Read the model definition and answer for the solid it produces. Units are mm, in the model's axes. A direction names the side the tool comes from. Give positions to 0.01 mm unless a question says otherwise; leave off trailing zeros. Order: outer loops, then holes, each group sorted by start corner. A loop starts at its lowest first (then second) coordinate and runs counter-clockwise, first axis right, second up. Notation, with made-up numbers: (-27, -22) - (2, -22) arc R24 ccw to (2, 10) - close; hole circle Ø10 at (71, -2). An arc over 180 degrees is marked (long way). Write item = value, one per line.
```python
from build123d import *

# Parameters (mm, degrees)
PAD_DEPTH         = 50
SKETCH001_R       = 20
POCKET_DEPTH      = 50.001
POCKET_DEPTH_BACK = 0.001
PAD001_DEPTH      = 10
SKETCH003_W       = 200
SKETCH003_H       = 125
PAD002_DEPTH      = 50
SKETCH004_W       = 25
SKETCH004_H       = 75
POCKET001_DEPTH   = 200.001
POCKET002_DEPTH   = 40


with BuildPart() as part:
    # Sketch → Pad (new body)
    with BuildSketch(Plane.XZ):
        with BuildLine():
            Line((-35, -35), (35, -35))
            Line((35, -35), (35, 0))
            ThreePointArc((35, 0), (0, 35), (-35, 0))
            Line((-35, 0), (-35, -35))
        make_face()
    extrude(amount=PAD_DEPTH)

    # Sketch001 (on Face6 of Pad) → Pocket (cut, two sides)
    with BuildSketch(Plane.XZ.offset(50)) as pocket_sk:
        Circle(SKETCH001_R)
    extrude(amount=-POCKET_DEPTH, mode=Mode.SUBTRACT)
    extrude(pocket_sk.sketch, amount=POCKET_DEPTH_BACK, mode=Mode.SUBTRACT)

    # Sketch002 (on Face5 of Pocket) → Pad001 (join)
    with BuildSketch(Plane.XZ.offset(50)):
        Polygon((35, -35), (95, -35), (22.707273, 26.634184), align=None)
    extrude(amount=-PAD001_DEPTH)

    # Sketch003 (on Face8 of Pad001) → Pad002 (join)
    with BuildSketch(Plane(origin=(0, 0, -35), x_dir=(1, 0, 0), z_dir=(0, 0, -1))):
        with Locations((65, -12.5)):
            Rectangle(SKETCH003_W, SKETCH003_H)
    extrude(amount=PAD002_DEPTH)

    # Sketch004 (on Face10 of Pad002) → Pocket001 (cut, through all)
    with BuildSketch(Plane(origin=(165, 0, 0), x_dir=(0, 0, 1), z_dir=(1, 0, 0))):
        with Locations((-72.5, -12.5)):
            Rectangle(SKETCH004_W, SKETCH004_H)
    extrude(amount=-POCKET001_DEPTH, mode=Mode.SUBTRACT)

    # Sketch005 (on Face16 of Pocket001) → Pocket002 (cut)
    with BuildSketch(Plane(origin=(85, 0, 0), x_dir=(0, 0, 1), z_dir=(1, 0, 0))):
        Polygon((-35, -55), (-35, -75), (-85, -75), align=None)
    extrude(amount=-POCKET002_DEPTH, mode=Mode.SUBTRACT)


solid = part.part
```
1. Section C-C (z = 3.5) is taken. Determine the outline of the cut face in (x, y).
Recorded:
outline = (-34.82, -50) - (-19.69, -50) - (-19.69, 0) - (-34.82, 0) - close; (19.69, -50) - (49.84, -50) - (49.84, -40) - (34.82, -40) - (34.82, 0) - (19.69, 0) - close
2. Flat-ended cylindrical pins translate along their axes: pin 1 (5 mm diameter, centred on y = 39, z = -64.5, fed in from -X); pin 2 (17.5 mm diameter, centred on y = -21, z = -11.5, fed in from +X); pin 3 (12 mm diameter, centred on x = 82.5, y = 19.5, fed in from +Z); pin 4 (4 mm diameter, centred on x = 62.5, y = 28.5, fed in from -Z). Find the tip coordinate at first contact, or state that the pin passes through.
Recorded:
pin_1 = through
pin_2 = 35
pin_3 = -35
pin_4 = -60
3. Straight lines are drawn through the part: L1, parallel to Z at x = 0, y = -15; L2, parallel to Y at x = 124, z = -61; L3, parallel to Z at x = 0, y = -33. For each, find the intervals that lie inside material, in ascending order. Write a range as [from, to].
Recorded:
L1 = [-60, -20], [20, 35]
L2 = [-50, -25], [50, 75]
L3 = [-85, -20], [20, 35]
4. Section B-B (x = 143) is taken. Determine the outline of the cut face in (y, z).
Recorded:
outline = (-50, -85) - (-25, -85) - (-25, -60) - (50, -60) - (50, -85) - (75, -85) - (75, -35) - (-50, -35) - close
5. For faces 4 (the face through (15, 0, -15)), 5 (the face through (66, 50, -73)), 6 (the face through (85, 69, -49)), 7 (the face through (56, -40, -20)), determine the directions among +Z, -Z, +X, -X, +Y, -Y from which every point of the face is accessible in a straight line to the end or side of a thin tool.
Recorded:
face_4 = +Z, +X, -X, +Y
face_5 = -Z, +X, -X
face_6 = +Z, +Y
face_7 = +Z, +X, +Y
6. Section A-A (y = -29.5) is taken. Determine the outline of the cut face in (x, z).
Recorded:
outline = (-35, -85) - (165, -85) - (165, -35) - (35, -35) - (35, 0) arc R35 ccw to (-35, 0) - close; hole circle Ø40 at (0, 0)
7. Determine the mould class of faces 1 (the face through (45, 69, -49)), 2 (the face through (66, 13, -60)), 3 (the face through (35, -20, -18)) for opening direction X: +X half, -X half, draft (parallel to the pull), parting line (faces both ways), or undercut.
Recorded:
face_1 = undercut
face_2 = draft
face_3 = +X half
8. Section D-D (x = 0) is taken. Determine the outline of the cut face in (y, z), and give its area (4 significant figures).
Recorded:
outline = (-50, -85) - (-25, -85) - (-25, -60) - (50, -60) - (50, -85) - (75, -85) - (75, -35) - (0, -35) - (0, -20) - (-50, -20) - close; (-50, 20) - (0, 20) - (0, 35) - (-50, 35) - close
area = 5,875 mm^2
